from build123d import *

# Parameters (mm, degrees)
F0_R     = 10.530807
F0_W     = 80.109231
F0_H     = 88.9
F1_DEPTH = 25.4


with BuildPart() as f1:
    # F0 (on Front) → F1 (new body)
    with BuildSketch(Plane.XZ):
        with BuildLine():
            ThreePointArc((47.640182, 31.529863), (7.585566, 71.584478), (-32.469049, 31.529863))
            Line((-32.469049, 31.529863), (47.640182, 31.529863))
        make_face()
        with Locations((7.585566, 53.75486)):
            Circle(F0_R, mode=Mode.SUBTRACT)
        with Locations((7.585566, -12.920137)):
            Rectangle(F0_W, F0_H)
    extrude(amount=F1_DEPTH)


solid = f1.part
Geometry check sheet. Reference: the model listing, model coordinates, mm. Coordinates: 2 decimals unless noted, no trailing zeros. Order: outer loops, then holes, each group sorted by start corner. A loop starts at its lowest first (then second) coordinate and runs counter-clockwise, first axis right, second up. Notation, with made-up numbers: (17.25, 56.25) - (23.25, 56.25) arc R25 cw to (23.25, 94.25) - close; hole circle Ø11 at (-4.5, -15). An arc over 180 degrees is marked (long way). Answer in a Markdown table with one row per item. Add a question column.
1) Cross-section at A-A, the plane z = 50.5. Record the cut outline in (x, y).
2) Cross-section at B-B, the plane y = -7.75. Record the cut outline in (x, z), then the cut area to 3 significant figures.
3) Material ranges on line 1 along Z through (x, y) = (8.5, -14.25); line 2 along Z through (x, y) = (1, -8.5); line 3 along Z through (x, y) = (-15.5, -16.5), recorded low to high. Write a range as [from, to].
4) Cross-section at C-C, the plane x = 8.5. Record the cut outline in (y, z).
5) Release check for a two-part mould opening along Z. For faces 1 (the flat face through (7, 0, 8)), 2 (the flat face through (7, -13, -57.37)), 3 (the cylindrical face through (8.466, -12.522, 71.575)), 4 (the cylindrical face through (12.44, -12.52, 44.41)) record: +Z half, -Z half, draft (parallel to the pull), parting line (faces both ways), or undercut.
6) Cross-section at D-D, the plane x = -6. Record the cut outline in (y, z).
7) Gauge pin test, flat ends, axial feed: P1, Ø24, axis at x = 7.59, z = 53.75, coming from the -Y side; P2, Ø3, axis at x = 28, y = -15, coming from the +Z side. Record the tip position at first contact, or that the pin passes through.
Check result:
| question | item | result |
|---|---|---|
| 1 | outline | (-27.69, -25.4) - (-2.43, -25.4) - (-2.43, 0) - (-27.69, 0) - close; (17.6, -25.4) - (42.86, -25.4) - (42.86, 0) - (17.6, 0) - close |
| 2 | outline | (-32.47, -57.37) - (47.64, -57.37) - (47.64, 31.53) arc R40.05 ccw to (-32.47, 31.53) - close; hole circle Ø21.06 at (7.59, 53.75) |
| 2 | area | 9,290 mm² |
| 3 | line 1 | z = [-57.37, 43.26], [64.25, 71.57] |
| 3 | line 2 | z = [-57.37, 45.54], [61.97, 71.04] |
| 3 | line 3 | z = [-57.37, 64.26] |
| 4 | outline | (-25.4, -57.37) - (0, -57.37) - (0, 43.26) - (-25.4, 43.26) - close; (-25.4, 64.25) - (0, 64.25) - (0, 71.57) - (-25.4, 71.57) - close |
| 5 | face 1 | draft |
| 5 | face 2 | -Z half |
| 5 | face 3 | +Z half |
| 5 | face 4 | undercut |
| 6 | outline | (-25.4, -57.37) - (0, -57.37) - (0, 69.21) - (-25.4, 69.21) - close |
| 7 | P1 | stops at y = -25.4 |
| 7 | P2 | stops at z = 66.84 |
